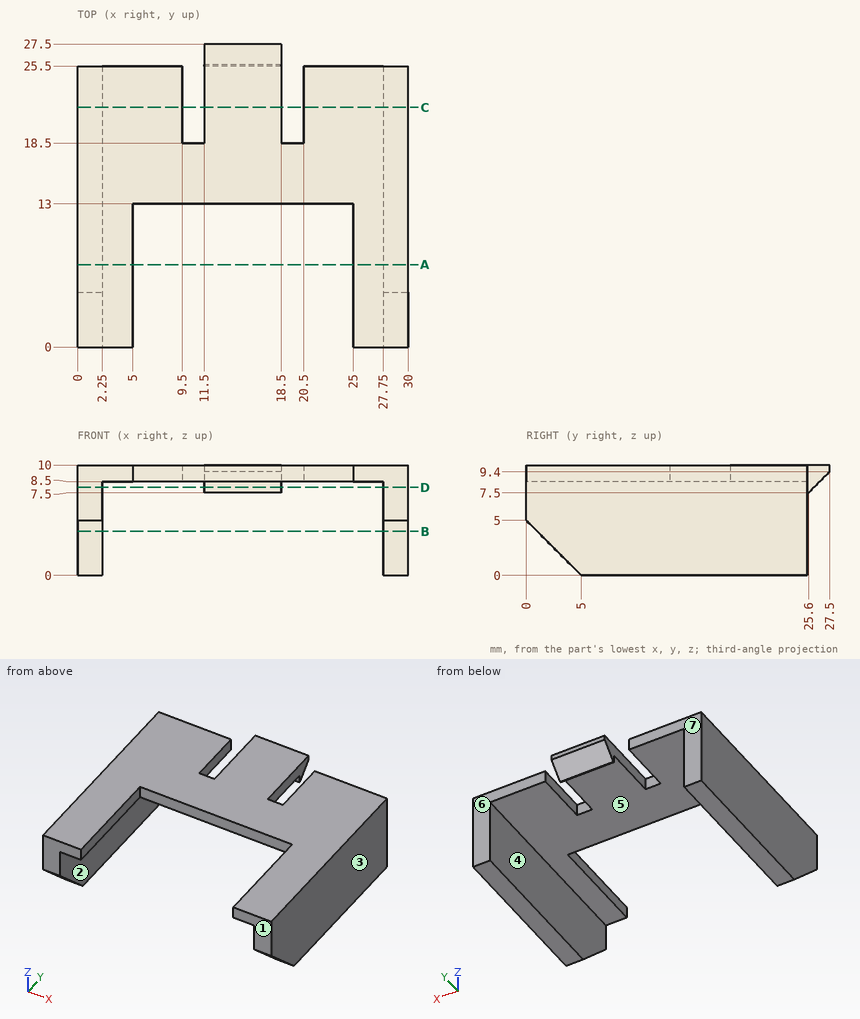
Source: three-view drawing plus pictorial views. Frame: mm from the lowest corner of the part. A direction names the side the tool comes from. Round coordinates to 2 decimals unless told otherwise and drop trailing zeros. Loops run counter-clockwise (first coordinate to the right, second up) from the corner with the lowest first, then second, coordinate; pieces in that order, holes last.
Q1. Section C-C on y = 21.75. Return loops of the section in (x, z), plus the area to 4 significant figures.
Q2. Pin query (flat end, axial travel): P1, Ø7.5, axis at x = 14, y = 10.5, coming from the -Z side; P2, Ø1.5, axis at x = 20.5, z = 9, coming from the -Y side; P3, Ø1.2, axis at x = 10.5, z = 9.5, coming from the +Y side; P4, Ø6, axis at x = 9, y = 3, coming from the -Z side. Return the tip coordinate at first contact, or that it passes through.
Q3. Section B-B on z = 4. Return loops of the section in (x, y).
Q4. Material intervals for L1, parallel to X at y = 25, z = 9.5; L2, parallel to X at y = 3.75, z = 3.75; L3, parallel to X at y = 7, z = 9, sorted ascending.
Q5. Section D-D on z = 8. Return loops of the section in (x, y), plus the area to 3 significant figures.
Q6. Section A-A on y = 7.5. Return loops of the section in (x, z), plus the area to 4 significant figures.
Q7. Access query for the marked faces 4, 5, 6 and 7. Directions: +Z, -Z, +X, -X, +Y, -Y. A direction counts if a zero-diameter tool reaches every point of the face in a straight line with its end or side. Return the directions, or none.
Q8. Pull-direction query (X, two-part tool) for the marked faces 1, 2 and 3; classes: released by +X, released by -X, zero draft, split by the parting line, or undercut.
Evaluation:
1. outline: (0, 0) - (2.25, 0) - (2.25, 8.5) - (9.5, 8.5) - (9.5, 10) - (0, 10) - close; (11.5, 8.5) - (18.5, 8.5) - (18.5, 10) - (11.5, 10) - close; (20.5, 8.5) - (27.75, 8.5) - (27.75, 0) - (30, 0) - (30, 10) - (20.5, 10) - close
1. area: 77.25 mm2
2. P1: stops at z = 8.5
2. P2: stops at y = 13
2. P3: stops at y = 18.5
2. P4: passes through
3. outline: (0, 1) - (2.25, 1) - (2.25, 25.5) - (0, 25.5) - close; (27.75, 1) - (30, 1) - (30, 25.5) - (27.75, 25.5) - close
4. L1: x = 0 to 9.5, 11.5 to 18.5, 20.5 to 30
4. L2: x = 0 to 2.25, 27.75 to 30
4. L3: x = 0 to 5, 25 to 30
5. outline: (0, 0) - (2.25, 0) - (2.25, 25.5) - (0, 25.5) - close; (11.5, 25.5) - (18.5, 25.5) - (18.5, 26.1) - (11.5, 26.1) - close; (27.75, 0) - (30, 0) - (30, 25.5) - (27.75, 25.5) - close
5. area: 119 mm2
6. outline: (0, 0) - (2.25, 0) - (2.25, 8.5) - (5, 8.5) - (5, 10) - (0, 10) - close; (25, 8.5) - (27.75, 8.5) - (27.75, 0) - (30, 0) - (30, 10) - (25, 10) - close
6. area: 53.25 mm2
7. face 4: -Z, +Y, -Y
7. face 5: -Z, -Y
7. face 6: +Z, -Z, +X, +Y
7. face 7: +Z, -Z, -X, +Y
8. face 1: zero draft
8. face 2: undercut
8. face 3: released by +X
